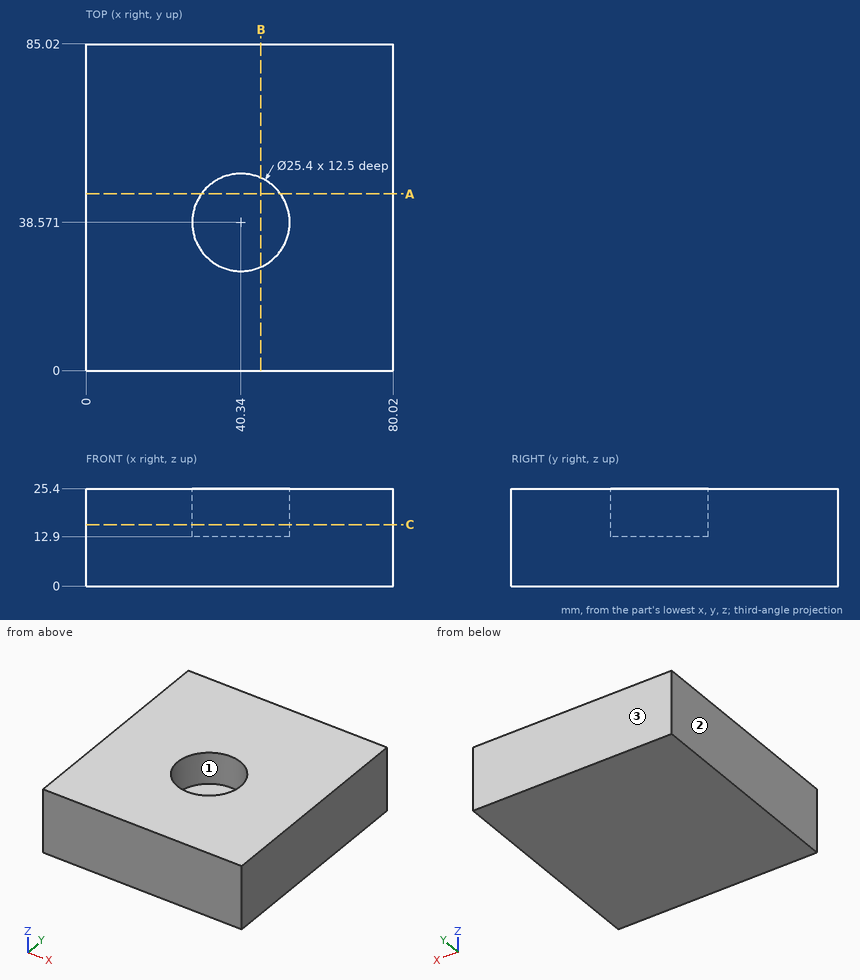
Source: three-view drawing plus pictorial views. Frame: mm from the lowest corner of the part. Give positions to 0.01 mm unless a question says otherwise; leave off trailing zeros. Order: outer loops, then holes, each group sorted by start corner. A loop starts at its lowest first (then second) coordinate and runs counter-clockwise, first axis right, second up. Notation, with made-up numbers: (-29, 18) -> (-19, 18) arc R18 ccw to (-19, 32) -> close; hole circle Ø7 at (71, 28). An arc over 180 degrees is marked (long way). Put each result on its own line as item: value.
Q1. Section B-B, the plane x = 45.5. Return loops of the section in (y, z) (1 decimal), then the cut area to 3 significant figures.
Here are the results:
outline: (0, 0) -> (85, 0) -> (85, 25.4) -> (50.2, 25.4) -> (50.2, 12.9) -> (27, 12.9) -> (27, 25.4) -> (0, 25.4) -> close
area: 1,870 mm^2
Q2. Section C-C, the plane z = 16. Return loops of the section in (x, y).
Here are the results:
outline: (0, 0) -> (80.02, 0) -> (80.02, 85.02) -> (0, 85.02) -> close; hole circle Ø25.4 at (40.34, 38.57)
Q3. Section A-A, the plane y = 46. Return loops of the section in (x, z).
Here are the results:
outline: (0, 0) -> (80.02, 0) -> (80.02, 25.4) -> (50.64, 25.4) -> (50.64, 12.9) -> (30.04, 12.9) -> (30.04, 25.4) -> (0, 25.4) -> close
Q4. Material intervals for L1, parallel to X at y = 49, z = 14 (1 decimal); L2, parallel to Z at x = 46, y = 38.5, sorted ascending.
Here are the results:
L1: x = 0 to 33.1, 47.6 to 80
L2: z = 0 to 12.9
Q5. Pin query (flat end, axial travel): pin 1 (2 mm diameter, centred on x = 30.5, y = 50, fed in from -Z); pin 2 (7.5 mm diameter, centred on x = 36.5, y = 37.5, fed in from +Z). Return the tip coordinate at first contact, or that it passes through.
Here are the results:
pin 1: stops at z = 0
pin 2: stops at z = 12.9
Q6. Draft query along X for the marked faces 1, 2 and 3. Return one class per face: released by +X, released by -X, zero draft, split by the parting line, or undercut.
Here are the results:
face 1: undercut
face 2: released by -X
face 3: zero draft
